```python
from build123d import *

# Parameters (mm, degrees)
SKETCH3_R           = 13.97
GEARBODY_DEPTH      = 3.175
TOOTHCUT_DEPTH      = 4.175
CIRPATTERN1_COUNT   = 9
BOREDIA_R           = 1.499997014
BORE_DEPTH          = 12700
BOSS_EXTRUDE1_DEPTH = 3.175
SKETCH5_R           = 0.508
CUT_EXTRUDE1_DEPTH  = 4.175


with BuildPart() as part:
    # Sketch3 → gearBody (new body)
    with BuildSketch(Plane.XY):
        Circle(SKETCH3_R)
    extrude(amount=GEARBODY_DEPTH)

    # Sketch2 → toothCut (cut, through all)
    with BuildSketch(Plane.XY):
        with BuildLine():
            ThreePointArc((7.654596591, -3.288775527), (7.788168987, -2.958600559), (7.907507119, -2.623018223))
            ThreePointArc((7.907507119, -2.623018223), (8.3519289, -2.073263372), (9.048439358, -1.952373766))
            ThreePointArc((9.048439358, -1.952373766), (13.146424788, -1.34364254), (15.979509974, 1.679214819))
            ThreePointArc((15.979509974, 1.679214819), (15.020212204, -5.705937852), (10.834165744, -11.865300419))
            ThreePointArc((10.834165744, -11.865300419), (10.7226862, -7.723850118), (8.062481966, -4.547790968))
            ThreePointArc((8.062481966, -4.547790968), (7.621913496, -3.994943305), (7.654596591, -3.288775527))
        make_face()
    toothcut = extrude(amount=TOOTHCUT_DEPTH, mode=Mode.SUBTRACT)

    # CirPattern1: toothCut ×9 about axis
    cirpattern1_axis = Axis((0, 0, 0), (0, 0, 1))
    for i in range(1, CIRPATTERN1_COUNT):
        add(toothcut.rotate(cirpattern1_axis, i * 360 / CIRPATTERN1_COUNT), mode=Mode.SUBTRACT)

    # boreDia → bore (cut, symmetric)
    with BuildSketch(Plane.XY):
        Circle(BOREDIA_R)
    extrude(amount=BORE_DEPTH, both=True, mode=Mode.SUBTRACT)

    # Sketch4 → Boss-Extrude1 (add)
    with BuildSketch(Plane(origin=(0, 0, 0), x_dir=(-1, 0, 0), z_dir=(0, 0, -1))):
        with BuildLine():
            Line((1.118029954, -1.000000032), (-1.118029954, -1.000000032))
            ThreePointArc((-1.118029954, -1.000000032), (0, -1.499997014), (1.118029954, -1.000000032))
        make_face()
    extrude(amount=-BOSS_EXTRUDE1_DEPTH)

    # Sketch5 → Cut-Extrude1 (cut, through all)
    with BuildSketch(Plane.XY.offset(3.175)):
        with Locations((-0.873392334, -0.554784988)):
            Circle(SKETCH5_R)
        with Locations((0.873392334, -0.554784988)):
            Circle(SKETCH5_R)
    extrude(amount=-CUT_EXTRUDE1_DEPTH, mode=Mode.SUBTRACT)


solid = part.part
```
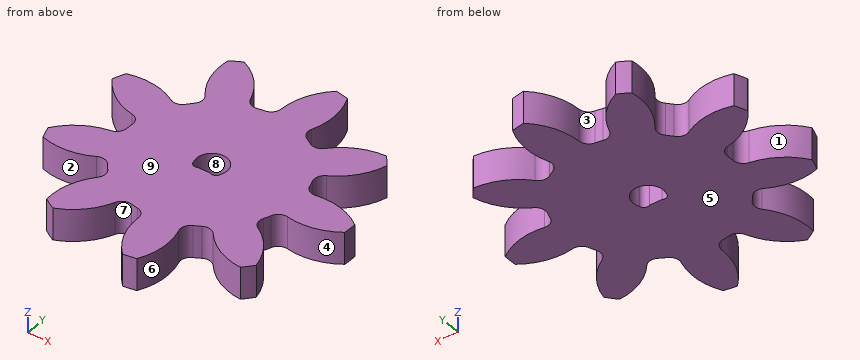
Can you work these out from the model? Positions are in its coordinate system, mm. Face numbers are marked on the shaded views. A direction names the side the tool comes from. Coordinates: 2 decimals unless noted, no trailing zeros. Loops run counter-clockwise (first coordinate to the right, second up) from the corner with the lowest first, then second, coordinate; pieces in that order, holes last. Notation, with made-up numbers: M 78,-36.75 L 100,-36.75 A24 cw 100,-26.75 Z; hole C 19,-10.75 d5. An arc over 180 degrees is marked long. Put each result on its own line as item: value. Start each with the question number.
(1) I need wall thicknesses on probe 1 along X at (y, z) = (0, 1.55); probe 2 along Y at (x, z) = (8.5, 1.5); probe 3 along X at (y, z) = (-11.5, 1.05). Which ranges of each line are inside material? Lowest first, please.
(2) Imagine slicing it at B-B on x = -9.75. List the corners of the cut face in (y, z) for me (3 decimals).
(3) Imagine slicing it at C-C on x = 12. List the corners of the cut face in (y, z) for me (3 decimals), and give its area (3 significant figures).
(4) We'd pull the mould along Y, two halves only. Please class the marked faces 6, 7, 8 and 9: +Y half, -Y half, draft (parallel to the pull), parting line (faces both ways), or undercut.
(5) Imagine slicing it at A-A on y = 7.75. List the corners of the cut face in (x, z) for me (3 decimals), and give its area (3 significant figures).
(6) Will these pins go through, and if not, where does the flat tip stop? pin 1 Ø1.5 at (x, y) = (-9.5, 9) entering from +Z; pin 2 Ø1.4 at (x, z) = (0.5, 1) entering from +Y; pin 3 Ø1.5 at (y, z) = (7, 2) entering from +X; pin 4 Ø1.5 at (x, z) = (-0.5, 2) entering from -Y.
(7) Which directions (+Z, -Z, +X, -X, +Y, -Y) give clear straight access to the entire face, cutting with the end or side of a thin tool? Please do the marked faces 1, 2, 3, 4 and 5.
Worked answers:
1. probe 1: x = -8.33 to -1.5, 1.5 to 13.97
1. probe 2: y = -9.28 to -4.83, -2 to 1.79, 4.51 to 8.95
1. probe 3: x = -7.72 to -5.15, 0.03 to 3.55
2. outline: M -5.373,0 L -1.383,0 L -1.383,3.175 L -5.373,3.175 Z; M 1.667,0 L 5.678,0 L 5.678,3.175 L 1.667,3.175 Z
3. outline: M -1.807,0 L 1.486,0 L 1.486,3.175 L -1.807,3.175 Z
3. area: 10.5 mm2
4. face 6: undercut
4. face 7: -Y half
4. face 8: undercut
4. face 9: draft
5. outline: M -6.527,0 L 3.543,0 L 3.543,3.175 L -6.527,3.175 Z; M 6.472,0 L 11.059,0 L 11.059,3.175 L 6.472,3.175 Z
5. area: 46.5 mm2
6. pin 1: passes through
6. pin 2: stops at y = 12.99
6. pin 3: stops at x = 11.06
6. pin 4: stops at y = -12.02
7. face 1: +Z, -Z, -X
7. face 2: +Z, -Z, -Y
7. face 3: +Z, -Z, +Y
7. face 4: +Z, -Z
7. face 5: -Z, +X, -X, +Y, -Y
